```python
from build123d import *

# Parameters (mm, degrees)
F1_DEPTH = 60
F3_DEPTH = 25


with BuildPart() as f1:
    # F0 (on Top) → F1 (new body)
    with BuildSketch(Plane.XY):
        Polygon((-54.709053, 31.494253), (-54.709053, -18.505747), (-39.709053, -18.505747), (-39.709053, 15.428343), (36.831179, 15.428343), (36.831179, -18.505747), (55.290947, -18.505747), (55.290947, 31.494253), align=None)
    extrude(amount=F1_DEPTH)

    # F2 (on face) → F3 (cut)
    with BuildSketch(Plane(origin=(-54.709053, 0, 0), x_dir=(0, -1, 0), z_dir=(-1, 0, 0))):
        Polygon((18.505747, 60), (-1.494253, 60), (18.505747, 50), align=None)
    extrude(amount=-F3_DEPTH, mode=Mode.SUBTRACT)


solid = f1.part
```
Could you check a few things on this model? Use its own coordinates, in mm. A direction names the side the tool comes from. Round coordinates to 2 decimals unless told otherwise and drop trailing zeros. Loops run counter-clockwise (first coordinate to the right, second up) from the corner with the lowest first, then second, coordinate; pieces in that order, holes last. Notation, with made-up numbers: (44.5, 44.25) -> (80.5, 44.25) arc R11 cw to (80.5, 51.25) -> close; hole circle Ø1 at (-38.75, -27). An arc over 180 degrees is marked (long way). One line per question, with ' | ' between items.
(1) If we section it at B-B on z = 41.5: List the corners of the cut face in (x, y) for me, and give its area (3 significant figures).
Model answer:
outline: (-54.71, -18.51) -> (-39.71, -18.51) -> (-39.71, 15.43) -> (36.83, 15.43) -> (36.83, -18.51) -> (55.29, -18.51) -> (55.29, 31.49) -> (-54.71, 31.49) -> close | area: 2,900 mm^2
(2) If we section it at D-D on y = -14: List the corners of the cut face in (x, z) for me, and give its area (3 significant figures).
Model answer:
outline: (-54.71, 0) -> (-39.71, 0) -> (-39.71, 52.25) -> (-54.71, 52.25) -> close; (36.83, 0) -> (55.29, 0) -> (55.29, 60) -> (36.83, 60) -> close | area: 1,890 mm^2
(3) If I drill on probe 1 along X at (y, z) = (14, 3); probe 2 along Y at (x, z) = (11, 31); probe 3 along X at (y, z) = (-14.5, 56), over which ranges is the centre line in solid material (lowest first)?
Model answer:
probe 1: x = -54.71 to -39.71, 36.83 to 55.29 | probe 2: y = 15.43 to 31.49 | probe 3: x = 36.83 to 55.29
(4) If we section it at C-C on x = 21: List the corners of the cut face in (y, z) for me, and give its area (3 significant figures).
Model answer:
outline: (15.43, 0) -> (31.49, 0) -> (31.49, 60) -> (15.43, 60) -> close | area: 964 mm^2
(5) Thinking about a two-plate mould opening in X: for faces 1 (the face through (-2, 15.428, 30)), 2 (the face through (46, -18.506, 30)), 3 (the face through (-54.709, 7, 30)), which applies, released by +X, released by -X, zero draft, split by the parting line, or undercut?
Model answer:
face 1: undercut | face 2: zero draft | face 3: released by -X
(6) If we section it at A-A on y = 13: List the corners of the cut face in (x, z) for me.
Model answer:
outline: (-54.71, 0) -> (-39.71, 0) -> (-39.71, 60) -> (-54.71, 60) -> close; (36.83, 0) -> (55.29, 0) -> (55.29, 60) -> (36.83, 60) -> close
(7) For faces 4 (the face through (-47.31, -8.37, 55.07)), 5 (the face through (0, 18, 0)), 6 (the face through (-39.709, -2, 30)), which set-ups out of +Z, -Z, +X, -X, +Y, -Y let a thin tool reach every point of the face, with its end or its side?
Model answer:
face 4: +Z, -X, -Y | face 5: -Z, +X, -X, +Y, -Y | face 6: +Z, -Z, -Y
(8) For pin 1 Ø10 at (x, y) = (-39.5, -7) entering from +Z; pin 2 Ø18 at (x, z) = (17, 18.5) entering from -Y, each with a flat end and sliding along its axis, tell me the tip position at first contact or that it passes through.
Model answer:
pin 1: stops at z = 58.25 | pin 2: stops at y = 15.43
